from build123d import *

# Parameters (mm, degrees)
SKETCH1_R           = 65.4431
SKETCH1_R_2         = 63.5
BOSS_EXTRUDE1_DEPTH = 863.6
CUT_EXTRUDE1_DEPTH  = 66.4431
CIRPATTERN1_COUNT   = 3


with BuildPart() as part:
    # Sketch1 → Boss-Extrude1 (new body)
    with BuildSketch(Plane(origin=(0, 0, 0), x_dir=(1, 0, 0), z_dir=(0, 1, 0))):
        Circle(SKETCH1_R)
        Circle(SKETCH1_R_2, mode=Mode.SUBTRACT)
    extrude(amount=BOSS_EXTRUDE1_DEPTH)

    # Sketch2 → Cut-Extrude1 (cut, through all)
    with BuildSketch(Plane.XY):
        with BuildLine():
            Line((7, 0), (7, 101.6))
            ThreePointArc((7, 101.6), (0, 108.6), (-7, 101.6))
            Line((-7, 101.6), (-7, 0))
            Line((-7, 0), (7, 0))
        make_face()
    cut_extrude1 = extrude(amount=-CUT_EXTRUDE1_DEPTH, mode=Mode.SUBTRACT)

    # CirPattern1: Cut-Extrude1 ×3 about axis
    cirpattern1_axis = Axis((0, 0, 0), (0, 1, 0))
    for i in range(1, CIRPATTERN1_COUNT):
        add(cut_extrude1.rotate(cirpattern1_axis, i * 360 / CIRPATTERN1_COUNT), mode=Mode.SUBTRACT)


solid = part.part
Verification items for the finished model (mm, model axes). Give positions to 0.01 mm unless a question says otherwise; leave off trailing zeros. Loops run counter-clockwise (first coordinate to the right, second up) from the corner with the lowest first, then second, coordinate; pieces in that order, holes last.
1) Depth check by flat-ended pin: pin 1 Ø8 at (x, y) = (-42.5, 168) entering from +Z; pin 2 Ø10 at (x, y) = (28.5, 197.5) entering from -Z; pin 3 Ø6 at (x, y) = (7.5, 124.5) entering from -Z. Enter the tip coordinate at first touch or a pass-through.
2) Thickness scan on line 1 along X through (y, z) = (570.5, 0); line 2 along Z through (x, y) = (2.5, 615.5). Record the ranges inside material, lowest first.
3) Draft check along Z on faces 1 (the flat face through (-56, 0, -33)), 2 (the cylindrical face through (62.42, 425.75, -19.66)), 3 (the cylindrical face through (-13.77, 425.75, 61.99)). Enter one of: pulls with the +Z half, pulls with the -Z half, needs draft (parallel to the pull), parting line crosses it, or undercut.
4) Sectioned sample at A-A, the plane z = 0. Enter the section's corners in (x, y).
5) Sectioned sample at B-B, the plane x = 19. Enter the section's corners in (y, z), then the cut area to 3 significant figures.
Answers:
1. pin 1: stops at z = 52.92
1. pin 2: stops at z = -61.08
1. pin 3: stops at z = -65.29
2. line 1: x = -65.44 to -63.5, 63.5 to 65.44
2. line 2: z = -65.4 to -63.45, 63.45 to 65.4
3. face 1: needs draft
3. face 2: parting line crosses it
3. face 3: undercut
4. outline: (-65.44, 0) - (-63.5, 0) - (-63.5, 863.6) - (-65.44, 863.6) - close; (63.5, 0) - (65.44, 0) - (65.44, 863.6) - (63.5, 863.6) - close
5. outline: (0, -62.62) - (863.6, -62.62) - (863.6, -60.59) - (0, -60.59) - close; (0, 60.59) - (863.6, 60.59) - (863.6, 62.62) - (0, 62.62) - close
5. area: 3,510 mm2
